```python
from build123d import *

# Parameters (mm, degrees)
SKETCH1_W           = 209.55
SKETCH1_H           = 80.01
BOSS_EXTRUDE1_DEPTH = 3.175
BOSS_EXTRUDE2_DEPTH = 3.175
SKETCH3_R           = 1.89865
CUT_EXTRUDE1_DEPTH  = 4.175
FILLET1_R           = 12.7
FILLET3_R           = 2.54
FILLET4_R           = 12.7


with BuildPart() as part:
    # Sketch1 → Boss-Extrude1 (new body)
    with BuildSketch(Plane(origin=(0, 0, 0), x_dir=(1, 0, 0), z_dir=(0, 1, 0))):
        Rectangle(SKETCH1_W, SKETCH1_H)
    extrude(amount=BOSS_EXTRUDE1_DEPTH)

    # Sketch2 → Boss-Extrude2 (add, through all)
    with BuildSketch(Plane(origin=(0, 3.175, 0), x_dir=(1, 0, 0), z_dir=(0, 1, 0))):
        with BuildLine():
            Line((104.775, 40.005), (136.525, 13.36358671))
            ThreePointArc((136.525, 13.36358671), (118.699650285, 5.41866207), (104.775, -8.255))
            Line((104.775, -8.255), (104.775, 40.005))
        make_face()
        with BuildLine():
            Line((-104.775, 40.005), (-136.525, 13.36358671))
            ThreePointArc((-136.525, 13.36358671), (-118.699650285, 5.41866207), (-104.775, -8.255))
            Line((-104.775, -8.255), (-104.775, 40.005))
        make_face()
    extrude(amount=-BOSS_EXTRUDE2_DEPTH)

    # Sketch3 → Cut-Extrude1 (cut, through all)
    with BuildSketch(Plane(origin=(0, 3.175, 0), x_dir=(1, 0, 0), z_dir=(0, 1, 0))):
        with Locations((36.5125, -20.955)):
            Circle(SKETCH3_R)
        with Locations((14.2875, -20.955)):
            Circle(SKETCH3_R)
        with Locations((-14.2875, -20.955)):
            Circle(SKETCH3_R)
        with Locations((-36.5125, -20.955)):
            Circle(SKETCH3_R)
        with Locations((36.5125, -1.905)):
            Circle(SKETCH3_R)
        with Locations((14.2875, -1.905)):
            Circle(SKETCH3_R)
        with Locations((-14.2875, -1.905)):
            Circle(SKETCH3_R)
        with Locations((-36.5125, -1.905)):
            Circle(SKETCH3_R)
    extrude(amount=-CUT_EXTRUDE1_DEPTH, mode=Mode.SUBTRACT)

    # Fillet1
    fillet1_edges = [part.edges().sort_by_distance(p)[0] for p in [
        (104.775, 1.5875, 8.255),
        (-104.775, 1.5875, 8.255),
    ]]
    fillet(fillet1_edges, radius=FILLET1_R)

    # Fillet3
    fillet3_edges = [part.edges().sort_by_distance(p)[0] for p in [
        (136.525, 1.5875, -13.36358671),
        (-136.525, 1.5875, -13.36358671),
        (104.775, 1.5875, 40.005),
        (-104.775, 1.5875, 40.005),
    ]]
    fillet(fillet3_edges, radius=FILLET3_R)

    # Fillet4
    fillet4_edges = [part.edges().sort_by_distance(p)[0] for p in [
        (-104.775, 1.5875, -40.005),
        (104.775, 1.5875, -40.005),
    ]]
    fillet(fillet4_edges, radius=FILLET4_R)


solid = part.part
```
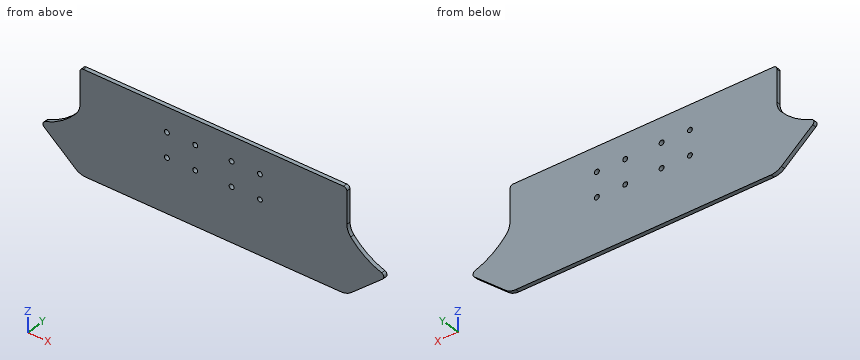
The model under review builds one solid part; all positions refer to its coordinate system, in mm. Round coordinates to 2 decimals unless told otherwise and drop trailing zeros. Loops run counter-clockwise (first coordinate to the right, second up) from the corner with the lowest first, then second, coordinate; pieces in that order, holes last. Notation, with made-up numbers: M 65.25,73 L 81.25,73 A20 ccw 81.25,101 Z; hole C 11.25,8 d7. An arc over 180 degrees is marked long. Write item = value, one per line.
Item 1: Insertion check: P1, Ø6, axis at x = -36.51, z = 1.9, coming from the -Y side; P2, Ø1, axis at y = 0.5, z = 7.5, coming from the +X side. Each pin has a flat end and moves straight along its axis. Give the tip position at first contact, or say it passes through.
Return value:
P1 = 0
P2 = 106.07
Item 2: Take a section at B-B on z = 31. Write out the cut boundary in (x, y) (3 decimals), then the cut area to 3 significant figures.
Return value:
outline = M -104.775,0 L 104.775,0 L 104.775,3.175 L -104.775,3.175 Z
area = 665 mm2
Item 3: For line 1 (Z direction, x = -36, y = 0.4) (3 decimals); line 2 (X direction, y = 0.8, z = 15.5) (3 decimals); line 3 (X direction, y = 0.4, z = -5), list the stretches that pass through material, from the lowest coordinate up. Write a range as [from, to].
Return value:
line_1 = [-40.005, 0.077], [3.733, 19.127], [22.783, 40.005]
line_2 = [-104.775, 104.775]
line_3 = [-118.09, 118.09]
Item 4: Take a section at C-C on z = -3. Write out the cut boundary in (x, y) (3 decimals).
Return value:
outline = M -115.416,0 L 115.416,0 L 115.416,3.175 L -115.416,3.175 Z
Item 5: Take a section at A-A on y = 1.6. State how many separate pieces and enclosed holes the cut face has, then the cut area to 3 significant figures.
Return value:
separate_pieces = 1
enclosed_holes = 8
area = 18,000 mm2
